For this review, take the finished solid that the model builds, in its own axes (mm). A direction names the side the tool comes from. Coordinates: 2 decimals unless noted, no trailing zeros. Write each loop counter-clockwise with the first axis right and the second up, starting at its lowest first coordinate (ties: lowest second). Pieces come first, ordered by that corner, then holes. Notation, with made-up numbers: M 58.25,78 L 95.25,78 A26 ccw 95.25,96 Z; hole C 86,61 d8. An arc over 180 degrees is marked long. One line per question, with ' | ' between items.
Solid Edge part; units mm, degrees
sketch "Sketch1" plane through (0, 0, 0) normal (0, -1, 0) x (1, 0, 0)
  line L0 (-5.0552, -8.6603) -> (4.9448, -8.6603)
  line L1 (4.9448, -8.6603) -> (9.9448, 0)
  line L2 (9.9448, 0) -> (4.9448, 8.6603)
  line L3 (4.9448, 8.6603) -> (-5.0552, 8.6603)
  line L4 (-5.0552, 8.6603) -> (-10.0552, 0)
  line L5 (-10.0552, 0) -> (-5.0552, -8.6603)
extrude "Protrusion1" add sketch "Sketch1" along normal mid plane 12
hole "Hole_1" at (0, -6, 0) direction (0, 1, 0) diameter 8.376 end up to next thread major 10 thread length 2
sketch "Sketch2" plane through (-0.0552, -6, 0) normal (0, -1, 0) x (1, 0, 0)
  line L0 (-14.8325, -1.4) -> (22.8043, -1.4)
  line L1 (22.8043, 1.4) -> (22.8043, -1.4)
  line L2 (-14.8325, 1.4) -> (22.8043, 1.4)
  line L3 (-14.8325, 1.4) -> (-14.8325, -1.4)
extrude "ExtrudedCutout_2" cut sketch "Sketch2" against normal blind 4
pattern_circular "Pattern1" count 3 over 360 about axis through (0, -6, 0) along (0, -1, 0) of "ExtrudedCutout_2"
1) We need section D-D on z = 3.75. State the section outline as (x, y) points.
Responses:
outline: M -7.89,-6 L -3.78,-6 L -3.78,-2 L -1.86,-2 L -1.86,6 L -7.89,6 Z; M 1.86,-2 L 3.78,-2 L 3.78,-6 L 7.78,-6 L 7.78,6 L 1.86,6 Z
2) To check wall thickness, follow line 1 along X through (y, z) = (-3, 4.75); line 2 along Z through (x, y) = (0, -3); line 3 along Y through (x, z) = (5.75, 1). State the ranges of each line that lie inside material, in increasing order. Write a range as [from, to].
Responses:
line 1: [-7.31, -4.36], [-1.13, 1.13], [4.36, 7.2] | line 2: [-8.66, -4.19], [4.19, 8.66] | line 3: [-2, 6]
3) Insertion check: pin 1 Ø5 at (y, z) = (3, -1) entering from +X; pin 2 Ø2 at (x, z) = (8, 0) entering from -Y; pin 3 Ø2 at (y, z) = (4.5, 2) entering from -X. Each pin has a flat end and moves straight along its axis. Give the tip position at first contact, or say it passes through.
Responses:
pin 1: x = 9.94 | pin 2: y = -2 | pin 3: x = -9.48
4) Machinability: for faces 1 (the flat face through (3, -2, -6)), 2 (the flat face through (7.48, 0.08, 4.27)), 3 (the flat face through (-7, -4, -1.4)), which of the approach directions +Z, -Z, +X, -X, +Y, -Y give a long, thin tool a straight path to every point of the face, cutting with its end or side? Answer none if there is none.
Responses:
face 1: -Y | face 2: +Z, +X, +Y, -Y | face 3: +X, -X, -Y
5) We need section A-A on x = 0. State the section outline as (y, z) points.
Responses:
outline: M -6,-8.66 L 6,-8.66 L 6,-4.19 L -6,-4.19 Z; M -6,4.19 L 6,4.19 L 6,8.66 L -6,8.66 Z
6) The part is to be moulded in two halves that separate along Z. For faces 4 (the flat face through (-6, -6, -4)), 5 (the flat face through (-4, -2, 6)), 6 (the flat face through (7.41, 0.08, -4.39)), say which applies: +Z half, -Z half, draft (parallel to the pull), parting line (faces both ways), or undercut.
Responses:
face 4: draft | face 5: undercut | face 6: -Z half
7) We need section B-B on y = 1.75. State the section outline as (x, z) points, then the cut area to 3 significant figures.
Responses:
outline: M -10.06,0 L -5.06,-8.66 L 4.94,-8.66 L 9.94,0 L 4.94,8.66 L -5.06,8.66 Z; hole C 0,0 d8.38 | area: 205 mm^2
8) We need section C-C on z = -1. State the section outline as (x, y) points, then the cut area to 3 significant figures.
Responses:
outline: M -9.48,-2 L -4.07,-2 L -4.07,6 L -9.48,6 Z; M 4.07,-2 L 9.37,-2 L 9.37,6 L 4.07,6 Z | area: 85.7 mm^2
